Model file for the job. Use its own axes, mm. Face numbers are marked on the shaded views. A direction names the side the tool comes from. Give positions to 0.01 mm unless a question says otherwise; leave off trailing zeros. Order: outer loops, then holes, each group sorted by start corner. A loop starts at its lowest first (then second) coordinate and runs counter-clockwise, first axis right, second up. Notation, with made-up numbers: (-13.75, -20) -> (-2.75, -20) arc R23 cw to (-2.75, -5) -> close; hole circle Ø3 at (-37.75, -34.75). An arc over 180 degrees is marked (long way). Use CSV: the item, a comma, the result in double quotes. Start each with the question number.
1. Cut at C-C on z = 0. List the corners of the cut face in (x, y).
2. Wall check: line 1 (Y direction, x = 0, z = 18.75); line 2 (Y direction, x = -0.5, z = 11); line 3 (X direction, y = 0, z = -13.5). Give the ranges that are in metal, low to high. Write a range as from..to.
3. Cut at A-A on z = 17.5. List the corners of the cut face in (x, y).
4. Drop flat-ended pins along their axis: pin 1 (1 mm diameter, centred on x = -1.5, z = 15.5, fed in from -Y); pin 2 (17 mm diameter, centred on x = 0, y = 0, fed in from +Z); pin 3 (1 mm diameter, centred on y = 11.5, z = -10, fed in from -X); pin 4 (2 mm diameter, centred on x = 13.75, y = 0, fed in from +Z). Give the stop position or say it passes through.
5. Cut at B-B on z = -15.5. List the corners of the cut face in (x, y).
6. Pull direction Y, two halves, no side cores. Call the marked faces 3, 4 and 5: released by +Y, released by -Y, zero draft, split by the parting line, or undercut.
7. 3-axis set-ups, long thin cutter, end or side, ignore diameter. For the marked faces 1 and 2: which of +Z, -Z, +X, -X, +Y, -Y reach the whole face in a straight line?
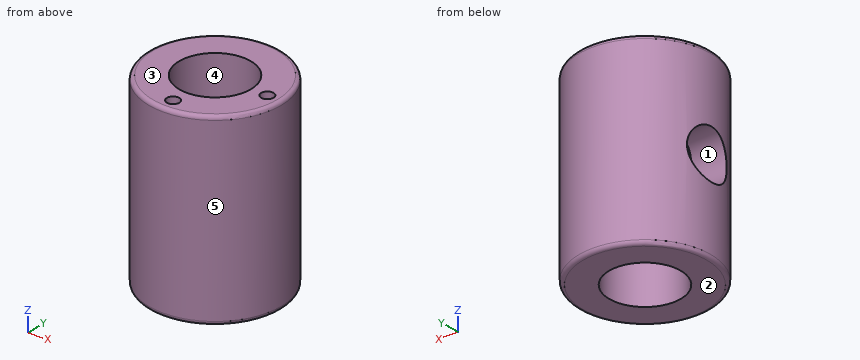
```python
from build123d import *

# Parameters (mm, degrees)
ESBO_O1_R                 = 17.5
ESBO_O1_R_2               = 9.5
RESSALTO_EXTRUS_O1_DEPTH  = 24.5
FILETE1_R                 = 1
ESBO_O2_R                 = 6.5
CORTE_EXTRUS_O1_DEPTH     = 35.824560299
FURO_ROSCADO_DE_M41_D     = 3.3
FURO_ROSCADO_DE_M41_DEPTH = 10
FURO_ROSCADO_DE_M41_TIP   = 0.991420021


with BuildPart() as part:
    # Esboço1 → Ressalto-extrusão1 (new, symmetric)
    with BuildSketch(Plane.XY):
        Circle(ESBO_O1_R)
        Circle(ESBO_O1_R_2, mode=Mode.SUBTRACT)
    extrude(amount=RESSALTO_EXTRUS_O1_DEPTH, both=True)

    # Filete1
    filete1_edges = [part.edges().sort_by_distance(p)[0] for p in [
        (-17.5, 0, -24.5),
        (-17.5, 0, 24.5),
    ]]
    fillet(filete1_edges, radius=FILETE1_R)

    # Esboço2 → Corte-extrusão1 (cut, through all)
    with BuildSketch(Plane(origin=(0, 0, 0), x_dir=(0, 0, -1), z_dir=(1, 0, 0))):
        Circle(ESBO_O2_R)
    extrude(amount=-CORTE_EXTRUS_O1_DEPTH, mode=Mode.SUBTRACT)

    # Furo roscado de M41
    with Locations(Plane.XY.offset(24.5)):
        with Locations((13.75, 0), (0, -13.75)):
            Hole(FURO_ROSCADO_DE_M41_D / 2, depth=FURO_ROSCADO_DE_M41_DEPTH)
            with Locations((0, 0, -(FURO_ROSCADO_DE_M41_DEPTH + FURO_ROSCADO_DE_M41_TIP / 2))):  # 118° drill point
                Cone(0, FURO_ROSCADO_DE_M41_D / 2, FURO_ROSCADO_DE_M41_TIP, mode=Mode.SUBTRACT)


solid = part.part
```
Verdict:
1,outline,"(-16.25, -6.5) arc R17.5 ccw (long way) to (-16.25, 6.5) -> (-6.93, 6.5) arc R9.5 cw (long way) to (-6.93, -6.5) -> close"
2,line 1,"-17.5..-15.4, -12.1..-9.5, 9.5..17.5"
2,line 2,"-17.49..-9.49, 9.49..17.49"
2,line 3,"-17.5..-9.5, 9.5..17.5"
3,outline,"circle Ø35 at (0, 0); hole circle Ø19 at (0, 0); hole circle Ø3.3 at (0, -13.75); hole circle Ø3.3 at (13.75, 0)"
4,pin 1,"y = -17.47"
4,pin 2,"through"
4,pin 3,"x = -13.61"
4,pin 4,"z = 14.11"
5,outline,"circle Ø35 at (0, 0); hole circle Ø19 at (0, 0)"
6,face 3,"zero draft"
6,face 4,"undercut"
6,face 5,"split by the parting line"
7,face 1,"-X"
7,face 2,"-Z, +X, -X, +Y, -Y"
